The figure shows three views and two pictorial views of one solid part (mm, origin at its lowest corner). Answer the questions. A direction names the side the tool comes from. Coordinates: 2 decimals unless noted, no trailing zeros. Order: outer loops, then holes, each group sorted by start corner. A loop starts at its lowest first (then second) coordinate and runs counter-clockwise, first axis right, second up. Notation, with made-up numbers: M 24,6.25 L 56,6.25 A17 cw 56,36.25 Z; hole C -36.5,73 d6. An arc over 180 degrees is marked long. Write item = value, one per line. Start each with the question number.
Q1. Find section C-C on x = 8. Give the vertices of the cut face in (y, z), and give its area (3 significant figures).
Q2. Straight lines are drawn through the part: line 1 along Y through (x, z) = (14, 10.25); line 2 along Y through (x, z) = (8.75, 1.6); line 3 along Z through (x, y) = (22, 3.25). For each, find the intervals that lie inside material, in ascending order.
Q3. Find section B-B on y = 14. Give the vertices of the cut face in (x, z), and give its area (3 significant figures).
Q4. Find section D-D on y = 7. Give the vertices of the cut face in (x, z).
Q5. Find section A-A on x = 14. Give the vertices of the cut face in (y, z).
Q6. A tool of negligible diameter and unlimited length cuts with its end or side. For the marked faces 1 and 2, from which of +Z, -Z, +X, -X, +Y, -Y can it reach the whole face along a straight path? Write none if from no direction.
Q7. Determine the mould class of the marked faces 3, 4 and 5 for opening direction Y: released by +Y, released by -Y, zero draft, split by the parting line, or undercut.
Q8. Each of these flat-tipped pins is pushed along its axis until it touches: P1, Ø10, axis at x = 21.5, y = 19.5, coming from the -Z side; P2, Ø2, axis at y = 16.5, z = 12.5, coming from the -X side; P3, Ø8, axis at y = 3.5, z = 12.5, coming from the +X side; P4, Ø6, axis at x = 18, z = 3.5, coming from the -Y side. Where does it stop, or does it pass through?
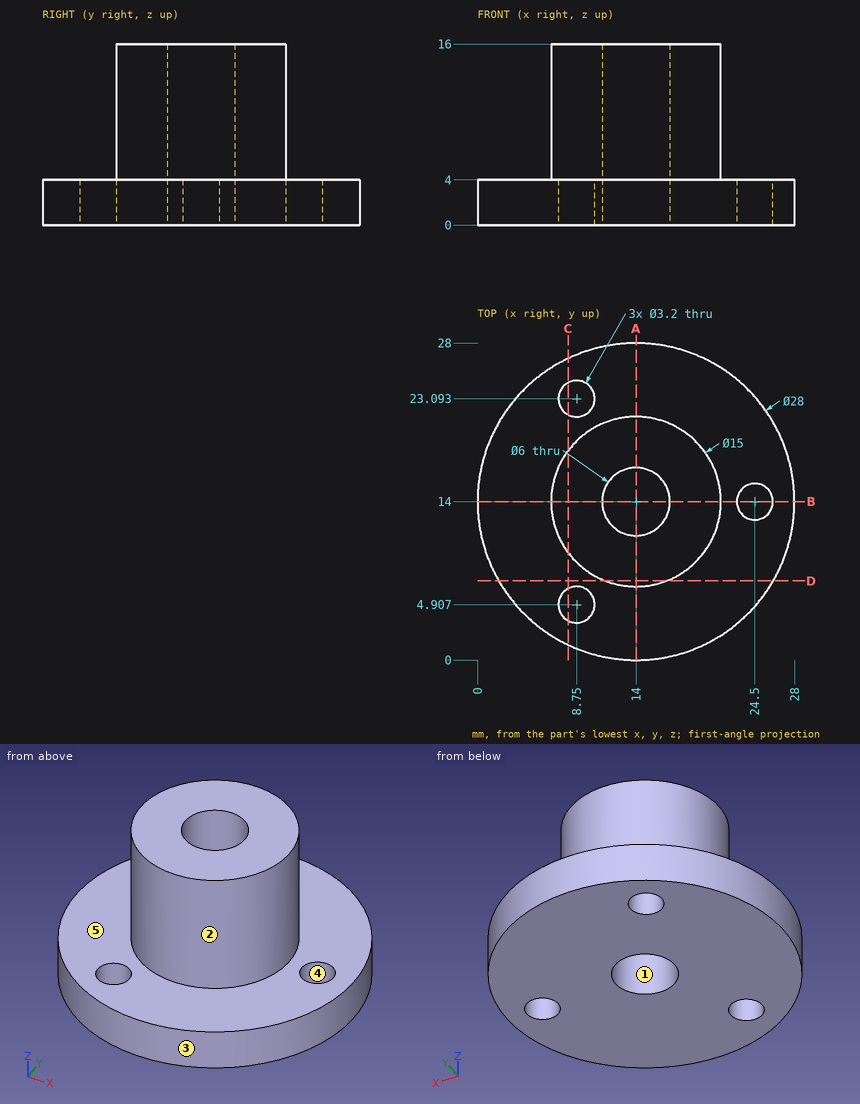
Findings below:
q1.outline = M 1.35,0 L 3.49,0 L 3.49,4 L 1.35,4 Z; M 6.32,0 L 21.68,0 L 21.68,4 L 18.5,4 L 18.5,16 L 9.5,16 L 9.5,4 L 6.32,4 Z; M 24.51,0 L 26.65,0 L 26.65,4 L 24.51,4 Z
q1.area = 187 mm^2
q2.line_1 = 6.5 to 11, 17 to 21.5
q2.line_2 = 1.02 to 3.31, 6.51 to 21.49, 24.69 to 26.98
q2.line_3 = 0 to 4
q3.outline = M 0,0 L 11,0 L 11,16 L 6.5,16 L 6.5,4 L 0,4 Z; M 17,0 L 22.9,0 L 22.9,4 L 21.5,4 L 21.5,16 L 17,16 Z; M 26.1,0 L 28,0 L 28,4 L 26.1,4 Z
q3.area = 183 mm^2
q4.outline = M 1.88,0 L 26.12,0 L 26.12,4 L 16.69,4 L 16.69,16 L 11.31,16 L 11.31,4 L 1.88,4 Z
q5.outline = M 0,0 L 11,0 L 11,16 L 6.5,16 L 6.5,4 L 0,4 Z; M 17,0 L 28,0 L 28,4 L 21.5,4 L 21.5,16 L 17,16 Z
q6.face_1 = +Z, -Z
q6.face_2 = +Z
q7.face_3 = split by the parting line
q7.face_4 = undercut
q7.face_5 = zero draft
q8.P1 = 0
q8.P2 = 6.65
q8.P3 = 17.74
q8.P4 = 0.04
